Can you work these out from the model? Positions are in its coordinate system, mm. Round coordinates to 2 decimals unless told otherwise and drop trailing zeros. Loops run counter-clockwise (first coordinate to the right, second up) from the corner with the lowest first, then second, coordinate; pieces in that order, holes last. Notation, with made-up numbers: (2, 73.5) -> (24, 73.5) arc R8 cw to (24, 87.5) -> close; hole circle Ø10 at (80.25, 72.25). An arc over 180 degrees is marked (long way). Use a Markdown table: item, result.
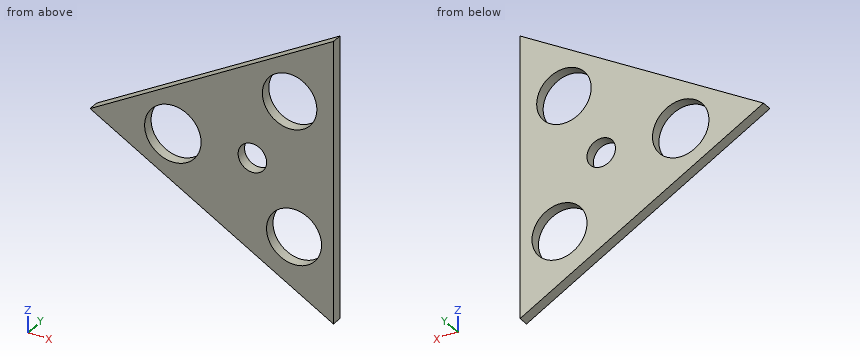
from build123d import *

# Parameters (mm, degrees)
F1_DEPTH  = 5
F2_R      = 13.153904
F4_DEPTH  = 51.562
F3_R      = 12.711179
F5_DEPTH  = 34.29
F6_R      = 12.830004
F7_DEPTH  = 49.276
F9_R      = 6.65
F10_DEPTH = 25.4


with BuildPart() as f1:
    # F0 (on Front) → F1 (new body)
    with BuildSketch(Plane.XZ):
        Polygon((37.830465, -65.524287), (37.830465, 65.524287), (-75.660929, 0), align=None)
    extrude(amount=F1_DEPTH)

    # F2 (on face) → F4 (cut)
    with BuildSketch(Plane.XZ.offset(5)):
        with Locations((-37.074074, 0)):
            Circle(F2_R)
    extrude(amount=-F4_DEPTH, mode=Mode.SUBTRACT)

    # F3 (on face) → F5 (cut)
    with BuildSketch(Plane.XZ.offset(5)):
        with Locations((17.382601, 31.523474)):
            Circle(F3_R)
    extrude(amount=-F5_DEPTH, mode=Mode.SUBTRACT)

    # F6 (on face) → F7 (cut)
    with BuildSketch(Plane.XZ.offset(5)):
        with Locations((19.439183, -30.693928)):
            Circle(F6_R)
    extrude(amount=-F7_DEPTH, mode=Mode.SUBTRACT)

    # F9 (on face) → F10 (cut)
    with BuildSketch(Plane.XZ.offset(5)):
        Circle(F9_R)
    extrude(amount=-F10_DEPTH, mode=Mode.SUBTRACT)


solid = f1.part
1. I want a section at D-D (x = 23.5). Please give me the cut outline in (y, z).
Answer sheet:
| item | result |
|---|---|
| outline | (-5, -57.25) -> (0, -57.25) -> (0, -42.86) -> (-5, -42.86) -> close; (-5, -18.52) -> (0, -18.52) -> (0, 20.38) -> (-5, 20.38) -> close; (-5, 42.67) -> (0, 42.67) -> (0, 57.25) -> (-5, 57.25) -> close |
2. I want a section at B-B (x = -44.5). Please give me the cut outline in (y, z).
Answer sheet:
| item | result |
|---|---|
| outline | (-5, -17.99) -> (0, -17.99) -> (0, -10.86) -> (-5, -10.86) -> close; (-5, 10.86) -> (0, 10.86) -> (0, 17.99) -> (-5, 17.99) -> close |
3. I want a section at A-A (z = -10). Please give me the cut outline in (x, y).
Answer sheet:
| item | result |
|---|---|
| outline | (-58.34, -5) -> (-45.62, -5) -> (-45.62, 0) -> (-58.34, 0) -> close; (-28.53, -5) -> (37.83, -5) -> (37.83, 0) -> (-28.53, 0) -> close |
4. Will these pins go through, and if not, where does the flat tip stop? pin 1 Ø21.5 at (x, z) = (0, 0) entering from +Y; pin 2 Ø2 at (y, z) = (-4.5, -17) entering from -X; pin 3 Ø3 at (y, z) = (-2.5, 44.5) entering from -X; pin 4 Ø3 at (y, z) = (-1, -22) entering from -X.
Answer sheet:
| item | result |
|---|---|
| pin 1 | stops at y = 0 |
| pin 2 | stops at x = -47.95 |
| pin 3 | stops at x = -1.18 |
| pin 4 | stops at x = -40.15 |
5. I want a section at C-C (y = -3.2). Please give me the cut outline in (x, z), plus the area to 3 significant figures.
Answer sheet:
| item | result |
|---|---|
| outline | (-75.66, 0) -> (37.83, -65.52) -> (37.83, 65.52) -> close; hole circle Ø26.31 at (-37.07, 0); hole circle Ø13.3 at (0, 0); hole circle Ø25.42 at (17.38, 31.52); hole circle Ø25.66 at (19.44, -30.69) |
| area | 5,730 mm² |
6. I need wall thicknesses on line 1 (X direction, y = -4.2, z = -0.5); line 2 (X direction, y = -4.4, z = 4.5); line 3 (Z direction, x = 13, y = -1). Which ranges of each line are inside material? Lowest first, please.
Answer sheet:
| item | result |
|---|---|
| line 1 | x = -74.79 to -50.22, -23.93 to -6.63, 6.63 to 37.83 |
| line 2 | x = -67.87 to -49.43, -24.71 to -4.9, 4.9 to 37.83 |
| line 3 | z = -51.19 to -41.79, -19.6 to 19.59, 43.46 to 51.19 |
